The model under review builds one solid part; all positions refer to its coordinate system, in mm. Face numbers are marked on the shaded views. A direction names the side the tool comes from. Coordinates: 2 decimals unless noted, no trailing zeros. Write each loop counter-clockwise with the first axis right and the second up, starting at its lowest first coordinate (ties: lowest second). Pieces come first, ordered by that corner, then holes. Notation, with made-up numbers: (27.5, 24.25) - (33.5, 24.25) arc R17 cw to (33.5, 49.25) - close; hole circle Ø7 at (69, 44.25). An arc over 180 degrees is marked (long way). Use one line per item in the form item = value. Start each with the question number.
```python
from build123d import *

# Parameters (mm, degrees)
SKETCH1_W               = 78.3
SKETCH1_H               = 14
BOSS_EXTRUDE1_DEPTH     = 2
SKETCH3_R               = 1.5
CUT_EXTRUDE2_DEPTH      = 1
CUT_EXTRUDE2_DEPTH_BACK = 3
SKETCH5_W               = 3
SKETCH5_H               = 3
BOSS_EXTRUDE2_DEPTH     = 2
SKETCH7_W               = 2
SKETCH7_H               = 14
BOSS_EXTRUDE3_DEPTH     = 8
CUT_EXTRUDE6_DEPTH      = 9.15
CUT_EXTRUDE6_DEPTH_BACK = 71.15


with BuildPart() as part:
    # Sketch1 → Boss-Extrude1 (new body)
    with BuildSketch(Plane(origin=(0, 0, 0), x_dir=(1, 0, 0), z_dir=(0, 1, 0))):
        with Locations((9.69964517, 3.832823468)):
            Rectangle(SKETCH1_W, SKETCH1_H)
    extrude(amount=BOSS_EXTRUDE1_DEPTH)

    # Sketch3 → Cut-Extrude2 (cut, two sides)
    with BuildSketch(Plane(origin=(0, 2, 0), x_dir=(1, 0, 0), z_dir=(0, 1, 0))) as cut_extrude2_sk:
        with Locations((-25.22535483, 0.832823468)):
            Circle(SKETCH3_R)
        with Locations((44.62464517, 0.832823468)):
            Circle(SKETCH3_R)
    extrude(amount=CUT_EXTRUDE2_DEPTH, mode=Mode.SUBTRACT)
    extrude(cut_extrude2_sk.sketch, amount=-CUT_EXTRUDE2_DEPTH_BACK, mode=Mode.SUBTRACT)

    # Sketch5 → Boss-Extrude2 (add)
    with BuildSketch(Plane.XZ):
        with Locations((-11.00035483, -9.332823468)):
            Rectangle(SKETCH5_W, SKETCH5_H)
        with Locations((30.39964517, -9.332823468)):
            Rectangle(SKETCH5_W, SKETCH5_H)
    extrude(amount=BOSS_EXTRUDE2_DEPTH)

    # Sketch7 → Boss-Extrude3 (add)
    with BuildSketch(Plane(origin=(0, 2, 0), x_dir=(1, 0, 0), z_dir=(0, 1, 0))):
        with Locations((39.69964517, 3.832823468)):
            Rectangle(SKETCH7_W, SKETCH7_H)
        with Locations((-20.30035483, 3.832823468)):
            Rectangle(SKETCH7_W, SKETCH7_H)
    extrude(amount=BOSS_EXTRUDE3_DEPTH)

    # Sketch9 → Cut-Extrude6 (cut, two sides)
    with BuildSketch(Plane.ZY.offset(21.30035483)) as cut_extrude6_sk:
        Polygon((3.167176532, 10), (3.167176532, 5), (-3.832823468, 10), align=None)
    extrude(amount=CUT_EXTRUDE6_DEPTH, mode=Mode.SUBTRACT)
    extrude(cut_extrude6_sk.sketch, amount=-CUT_EXTRUDE6_DEPTH_BACK, mode=Mode.SUBTRACT)


solid = part.part
```
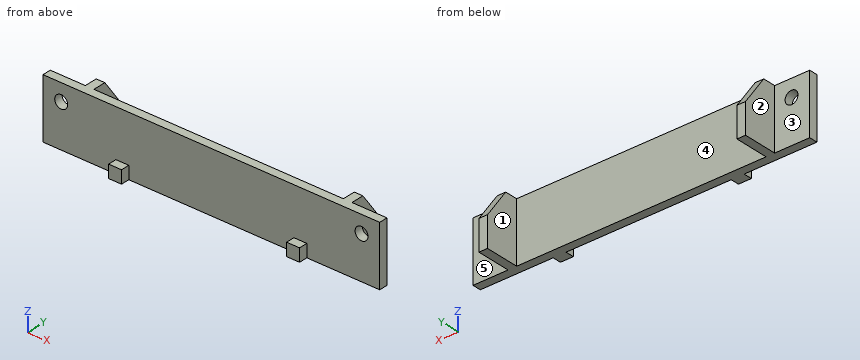
1. For L1, parallel to X at y = 5.75, z = -5.5; L2, parallel to Y at x = 15, z = -9.75; L3, parallel to Z at x = 40, y = 8.5, list the stretches that pass through material, from the lowest coordinate up.
2. Take a section at B-B (z = -9). State the section outline as (x, y) points, plus the area to 3 significant figures.
3. Take a section at A-A (y = -1). State the section outline as (x, z) points, plus the area to 3 significant figures.
4. The part is to be moulded in two halves that separate along X. For the marked faces 1, 2 and 3, say which applies: released by +X, released by -X, zero draft, split by the parting line, or undercut.
5. Take a section at C-C (x = -11.5). State the section outline as (y, z) points.
6. Take a section at D-D (y = 6.25). State the section outline as (x, z) points.
7. For the marked faces 4 and 5, list the 3-axis set-ups (+Z, -Z, +X, -X, +Y, -Y) from which the entire face can be reached by the end or side of a thin tool; tool diameter is ignored.
8. For P1, Ø2.5, axis at y = 4.5, z = -7, coming from the +X side; P2, Ø6.5, axis at x = 44, z = -5, coming from the +Y side; P3, Ø1, axis at x = 29.5, y = -1, coming from the +Z side, all flat-tipped, find the tip position at first contact; note any pin that passes through.
Returned:
q1.L1 = -21.3 to -19.3, 38.7 to 40.7
q1.L2 = 0 to 2
q1.L3 = -10.83 to -1.73
q2.outline = (-29.45, 0) - (-12.5, 0) - (-12.5, -2) - (-9.5, -2) - (-9.5, 0) - (28.9, 0) - (28.9, -2) - (31.9, -2) - (31.9, 0) - (48.85, 0) - (48.85, 2) - (40.7, 2) - (40.7, 10) - (38.7, 10) - (38.7, 2) - (-19.3, 2) - (-19.3, 10) - (-21.3, 10) - (-21.3, 2) - (-29.45, 2) - close
q2.area = 201 mm²
q3.outline = (-12.5, -10.83) - (-9.5, -10.83) - (-9.5, -7.83) - (-12.5, -7.83) - close; (28.9, -10.83) - (31.9, -10.83) - (31.9, -7.83) - (28.9, -7.83) - close
q3.area = 18.0 mm²
q4.face_1 = undercut
q4.face_2 = released by -X
q4.face_3 = zero draft
q5.outline = (-2, -10.83) - (2, -10.83) - (2, 3.17) - (0, 3.17) - (0, -7.83) - (-2, -7.83) - close
q6.outline = (-21.3, -10.83) - (-19.3, -10.83) - (-19.3, 1.42) - (-21.3, 1.42) - close; (38.7, -10.83) - (40.7, -10.83) - (40.7, 1.42) - (38.7, 1.42) - close
q7.face_4 = +Z, -Z, +Y
q7.face_5 = +Z, -Z, +X, +Y
q8.P1 = 40.7
q8.P2 = 2
q8.P3 = -7.83
